Geometry: final body of the model. Coordinates: model frame, mm. Give positions to 0.01 mm unless a question says otherwise; leave off trailing zeros. Write each loop counter-clockwise with the first axis right and the second up, starting at its lowest first coordinate (ties: lowest second). Pieces come first, ordered by that corner, then holes.
Q1. Cut plane A-A on x = 0. Return the cut outline in (y, z), plus the area to 3 significant figures.
Q2. Pin query (flat end, axial travel): pin 1 (1.2 mm diameter, centred on x = -12.5, z = -1.5, fed in from -Y); pin 2 (0.5 mm diameter, centred on y = 0.5, z = 13.5, fed in from -X); pin 3 (2 mm diameter, centred on x = 5.5, z = -4.5, fed in from +Y); pin 4 (0.8 mm diameter, centred on y = 0.5, z = 13.5, fed in from +X). Return the tip coordinate at first contact, or that it passes through.
Q3. Cut plane B-B on y = 1.95. Return the cut outline in (x, z), plus the area to 3 significant figures.
Q4. Line query: L1, parallel to X at y = 1, z = 0; L2, parallel to Z at x = -2.5, y = 0.95; L3, parallel to Y at x = -7, z = 10. Output: solid intervals per line, ascending.
```python
from build123d import *

# Parameters (mm, degrees)
SKETCH1_R           = 16
SKETCH1_W           = 2
SKETCH1_H           = 3
SKETCH1_R_2         = 10
BOSS_EXTRUDE3_DEPTH = 1
SKETCH2_R           = 16
SKETCH2_R_2         = 10
BOSS_EXTRUDE4_DEPTH = 1.5


with BuildPart() as part:
    # Sketch1 → Boss-Extrude3 (new body)
    with BuildSketch(Plane(origin=(0, 0, 0), x_dir=(1, 0, 0), z_dir=(0, 1, 0))):
        with Locations(Location((0, 0, 0), (0, 0, 270))):
            Circle(SKETCH1_R)
        Polygon((3.992867118, 13.97522852), (3.369132045, 11.040785718), (1.412836844, 11.456609099), (2.036571916, 14.391051901), align=None, mode=Mode.SUBTRACT)
        with Locations((0, 13)):
            Rectangle(SKETCH1_W, SKETCH1_H, mode=Mode.SUBTRACT)
        Polygon((6.811226782, 12.839672493), (5.591016853, 10.09903612), (3.763925938, 10.912509406), (4.984135867, 13.653145779), align=None, mode=Mode.SUBTRACT)
        Polygon((-2.036571916, 14.391051901), (-1.412836844, 11.456609099), (-3.369132045, 11.040785718), (-3.992867118, 13.97522852), align=None, mode=Mode.SUBTRACT)
        Polygon((9.331903153, 11.142961166), (7.568547396, 8.715910183), (5.950513407, 9.891480688), (7.713869164, 12.318531671), align=None, mode=Mode.SUBTRACT)
        Polygon((-4.984135867, 13.653145779), (-3.763925938, 10.912509406), (-5.591016853, 10.09903612), (-6.811226782, 12.839672493), align=None, mode=Mode.SUBTRACT)
        Polygon((-9.331903153, -11.142961166), (-7.568547396, -8.715910183), (-5.950513407, -9.891480688), (-7.713869164, -12.318531671), align=None, mode=Mode.SUBTRACT)
        Polygon((-11.444730576, -8.959248967), (-9.215296099, -6.951857148), (-7.877034887, -8.438146799), (-10.106469363, -10.445538618), align=None, mode=Mode.SUBTRACT)
        Polygon((-6.811226782, -12.839672493), (-5.591016853, -10.09903612), (-3.763925938, -10.912509406), (-4.984135867, -13.653145779), align=None, mode=Mode.SUBTRACT)
        with Locations((0, -13)):
            Rectangle(SKETCH1_W, SKETCH1_H, mode=Mode.SUBTRACT)
        Polygon((-1.412836844, -11.456609099), (-2.036571916, -14.391051901), (-3.992867118, -13.97522852), (-3.369132045, -11.040785718), align=None, mode=Mode.SUBTRACT)
        Polygon((-13.057368355, -6.383974596), (-10.459292144, -4.883974596), (-9.459292144, -6.616025404), (-12.057368355, -8.116025404), align=None, mode=Mode.SUBTRACT)
        Polygon((-14.099336481, -3.529689902), (-11.246166932, -2.602638919), (-10.628132943, -4.504751952), (-13.481302492, -5.431802935), align=None, mode=Mode.SUBTRACT)
        Polygon((-14.525095946, -0.521140822), (-11.54153026, -0.207555432), (-11.332473333, -2.196599223), (-14.31603902, -2.510184613), align=None, mode=Mode.SUBTRACT)
        Polygon((2.036571916, -14.391051901), (1.412836844, -11.456609099), (3.369132045, -11.040785718), (3.992867118, -13.97522852), align=None, mode=Mode.SUBTRACT)
        Polygon((4.984135867, -13.653145779), (3.763925938, -10.912509406), (5.591016853, -10.09903612), (6.811226782, -12.839672493), align=None, mode=Mode.SUBTRACT)
        Polygon((7.713869164, -12.318531671), (5.950513407, -9.891480688), (7.568547396, -8.715910183), (9.331903153, -11.142961166), align=None, mode=Mode.SUBTRACT)
        Polygon((10.106469363, -10.445538618), (7.877034887, -8.438146799), (9.215296099, -6.951857148), (11.444730576, -8.959248967), align=None, mode=Mode.SUBTRACT)
        Polygon((12.057368355, -8.116025404), (9.459292144, -6.616025404), (10.459292144, -4.883974596), (13.057368355, -6.383974596), align=None, mode=Mode.SUBTRACT)
        Polygon((13.481302492, -5.431802935), (10.628132943, -4.504751952), (11.246166932, -2.602638919), (14.099336481, -3.529689902), align=None, mode=Mode.SUBTRACT)
        Polygon((14.31603902, -2.510184613), (11.332473333, -2.196599223), (11.54153026, -0.207555432), (14.525095946, -0.521140822), align=None, mode=Mode.SUBTRACT)
        Polygon((-14.31603902, 2.510184613), (-11.332473333, 2.196599223), (-11.54153026, 0.207555432), (-14.525095946, 0.521140822), align=None, mode=Mode.SUBTRACT)
        Polygon((-13.481302492, 5.431802935), (-10.628132943, 4.504751952), (-11.246166932, 2.602638919), (-14.099336481, 3.529689902), align=None, mode=Mode.SUBTRACT)
        with Locations(Location((0, 0, 0), (0, 0, 270))):
            Circle(SKETCH1_R_2, mode=Mode.SUBTRACT)
        Polygon((-12.057368355, 8.116025404), (-9.459292144, 6.616025404), (-10.459292144, 4.883974596), (-13.057368355, 6.383974596), align=None, mode=Mode.SUBTRACT)
        Polygon((-10.106469363, 10.445538618), (-7.877034887, 8.438146799), (-9.215296099, 6.951857148), (-11.444730576, 8.959248967), align=None, mode=Mode.SUBTRACT)
        Polygon((-7.713869164, 12.318531671), (-5.950513407, 9.891480688), (-7.568547396, 8.715910183), (-9.331903153, 11.142961166), align=None, mode=Mode.SUBTRACT)
        Polygon((14.525095946, 0.521140822), (11.54153026, 0.207555432), (11.332473333, 2.196599223), (14.31603902, 2.510184613), align=None, mode=Mode.SUBTRACT)
        Polygon((14.099336481, 3.529689902), (11.246166932, 2.602638919), (10.628132943, 4.504751952), (13.481302492, 5.431802935), align=None, mode=Mode.SUBTRACT)
        Polygon((7.877034887, 8.438146799), (10.106469363, 10.445538618), (11.444730576, 8.959248967), (9.215296099, 6.951857148), align=None, mode=Mode.SUBTRACT)
        Polygon((13.057368355, 6.383974596), (10.459292144, 4.883974596), (9.459292144, 6.616025404), (12.057368355, 8.116025404), align=None, mode=Mode.SUBTRACT)
    extrude(amount=BOSS_EXTRUDE3_DEPTH)

    # Sketch2 → Boss-Extrude4 (add)
    with BuildSketch(Plane(origin=(0, 1, 0), x_dir=(1, 0, 0), z_dir=(0, 1, 0))):
        with Locations(Location((0, 0, 0), (0, 0, 270))):
            Circle(SKETCH2_R)
        with Locations(Location((0, 0, 0), (0, 0, 270))):
            Circle(SKETCH2_R_2, mode=Mode.SUBTRACT)
    extrude(amount=BOSS_EXTRUDE4_DEPTH)


solid = part.part
```
Data:
1. outline: (0, -16) - (2.5, -16) - (2.5, -10) - (0, -10) - (0, -11.5) - (1, -11.5) - (1, -14.5) - (0, -14.5) - close; (0, 10) - (2.5, 10) - (2.5, 16) - (0, 16) - (0, 14.5) - (1, 14.5) - (1, 11.5) - (0, 11.5) - close
1. area: 24.0 mm2
2. pin 1: stops at y = 1
2. pin 2: stops at x = -8.97
2. pin 3: passes through
2. pin 4: stops at x = 9.19
3. outline: circle Ø32 at (0, 0); hole circle Ø20 at (0, 0)
3. area: 490 mm2
4. L1: x = -16 to -10, 10 to 16
4. L2: z = -15.8 to -14.29, -11.23 to -9.68, 9.68 to 11.23, 14.29 to 15.8
4. L3: y = 1 to 2.5
